from build123d import *

# Parameters (mm, degrees)
BOSS_EXTRUDE1_DEPTH     = 20
CUT_EXTRUDE1_DEPTH      = 142.509716981
CUT_EXTRUDE1_DEPTH_BACK = 20
SKETCH2_W               = 20
SKETCH2_H               = 20
SKETCH2_H_2             = 40


with BuildPart() as part:
    # Sketch1 → Boss-Extrude1 (new body)
    with BuildSketch(Plane.XY):
        Polygon((0, 0), (60, 0), (80, 20), (80, 115), (56, 115), (-10, 97.3153533), (-10, 17.3153533), align=None)
    extrude(amount=BOSS_EXTRUDE1_DEPTH)

    # Sketch2 → Cut-Extrude1 (cut, two sides: drawn at the far end of the back side and taken through both)
    with BuildSketch(Plane.XY.offset(20).offset(-CUT_EXTRUDE1_DEPTH_BACK)):
        with Locations((68, 105)):
            Rectangle(SKETCH2_W, SKETCH2_H)
        Polygon((54, 93.758578007), (54, 114.464101615), (-8, 97.851251684), (-8, 77.145728076), align=None)
        with Locations((70, 45)):
            Rectangle(SKETCH2_W, SKETCH2_H_2)
    extrude(amount=CUT_EXTRUDE1_DEPTH + CUT_EXTRUDE1_DEPTH_BACK, mode=Mode.SUBTRACT)


solid = part.part
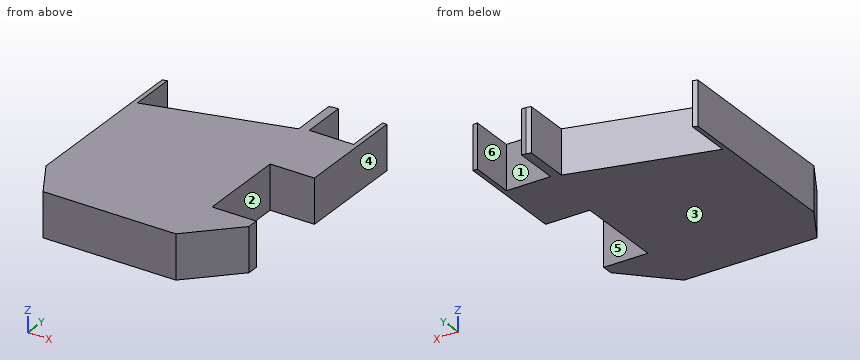
Could you check a few things on this model? Use its own coordinates, in mm. Face numbers are marked on the shaded views. A direction names the side the tool comes from. Round coordinates to 2 decimals unless told otherwise and drop trailing zeros. Write each loop counter-clockwise with the first axis right and the second up, starting at its lowest first coordinate (ties: lowest second). Pieces come first, ordered by that corner, then holes. Notation, with made-up numbers: (19, -25.75) -> (46, -25.75) arc R22 ccw to (46, -13.75) -> close; hole circle Ø4 at (75.5, 8.5). An arc over 180 degrees is marked (long way). Use a Markdown table: item, result.
1. If we section it at A-A (x = 68): List the corners of the cut face in (y, z) for me, then the cut area to 3 significant figures.
Answer key:
| item | result |
|---|---|
| outline | (8, 0) -> (25, 0) -> (25, 20) -> (8, 20) -> close; (65, 0) -> (95, 0) -> (95, 20) -> (65, 20) -> close |
| area | 940 mm^2 |
2. We'd pull the mould along X, two halves only. Please class the marked faces 4, 5 and 6: +X half, -X half, draft (parallel to the pull), parting line (faces both ways), or undercut.
Answer key:
| item | result |
|---|---|
| face 4 | +X half |
| face 5 | draft |
| face 6 | undercut |
3. Please list where these lines run through material, in increasing order: probe 1 along X at (y, z) = (107.5, 16); probe 2 along Y at (x, z) = (67, 12); probe 3 along X at (y, z) = (36, 6.75).
Answer key:
| item | result |
|---|---|
| probe 1 | x = 54 to 58, 78 to 80 |
| probe 2 | y = 7 to 25, 65 to 95 |
| probe 3 | x = -10 to 60 |
4. Which directions (+Z, -Z, +X, -X, +Y, -Y) give clear straight access to the entire face, cutting with the end or side of a thin tool? Please do the marked faces 1, 2 and 3.
Answer key:
| item | result |
|---|---|
| face 1 | +Z, -Z, +Y |
| face 2 | +Z, -Z, +X |
| face 3 | -Z, +X, -X, +Y, -Y |
5. If we section it at C-C (z = 9.75): List the corners of the cut face in (x, y) for me.
Answer key:
| item | result |
|---|---|
| outline | (-10, 17.32) -> (0, 0) -> (60, 0) -> (80, 20) -> (80, 25) -> (60, 25) -> (60, 65) -> (80, 65) -> (80, 115) -> (78, 115) -> (78, 95) -> (58, 95) -> (58, 115) -> (56, 115) -> (54, 114.46) -> (54, 93.76) -> (-8, 77.15) -> (-8, 97.85) -> (-10, 97.32) -> close |
6. For pin 1 Ø5 at (x, y) = (69, 64) entering from -Z; pin 2 Ø6 at (x, z) = (74.5, 8.5) entering from -Y; pin 3 Ø12 at (x, z) = (4, 10) entering from +Y; pin 4 Ø10 at (y, z) = (108.5, 7.5) entering from -X, each with a flat end and sliding along its axis, tell me the tip position at first contact or that it passes through.
Answer key:
| item | result |
|---|---|
| pin 1 | stops at z = 0 |
| pin 2 | stops at y = 11.5 |
| pin 3 | stops at y = 81.97 |
| pin 4 | stops at x = 54 |
7. If we section it at B-B (y = 100): List the corners of the cut face in (x, z) for me, then the cut area to 3 significant figures.
Answer key:
| item | result |
|---|---|
| outline | (54, 0) -> (58, 0) -> (58, 20) -> (54, 20) -> close; (78, 0) -> (80, 0) -> (80, 20) -> (78, 20) -> close |
| area | 120 mm^2 |
8. If we section it at D-D (y = 60): List the corners of the cut face in (x, z) for me.
Answer key:
| item | result |
|---|---|
| outline | (-10, 0) -> (60, 0) -> (60, 20) -> (-10, 20) -> close |
